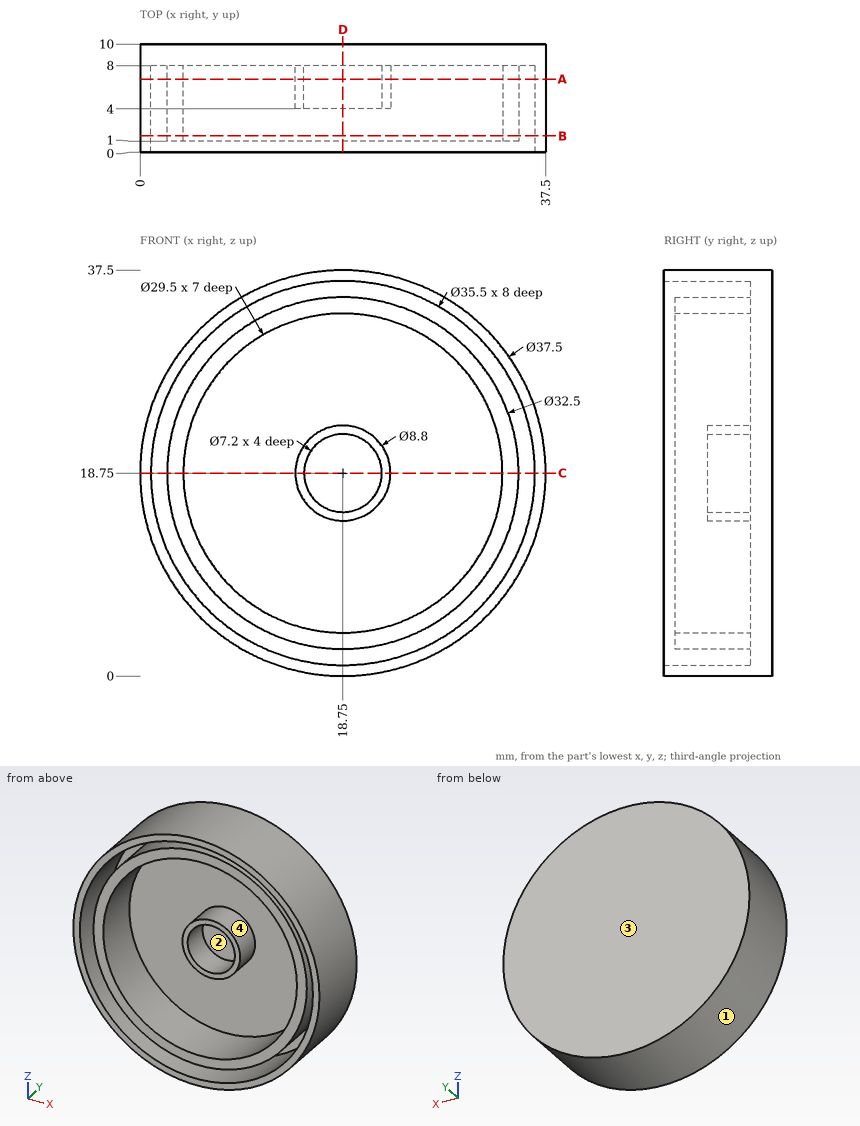
The drawing under review shows one solid part. Ordinate dimensions are in mm from its lowest x, y, z. Coordinates: 2 decimals unless noted, no trailing zeros. Write each loop counter-clockwise with the first axis right and the second up, starting at its lowest first coordinate (ties: lowest second). Pieces come first, ordered by that corner, then holes. Notation, with made-up numbers: M 62,-18 L 103,-18 A25 ccw 103,-1 Z; hole C 81,44.5 d5. An arc over 180 degrees is marked long. Answer as a JSON object with one key per item and string values.
Item 1: Add section D-D, the plane x = 18.75. Give the boundary of the cut face in (y, z).
Outcome:
{"outline": "M 0,0 L 10,0 L 10,37.5 L 0,37.5 L 0,36.5 L 8,36.5 L 8,35 L 1,35 L 1,33.5 L 8,33.5 L 8,23.15 L 4,23.15 L 4,22.35 L 8,22.35 L 8,15.15 L 4,15.15 L 4,14.35 L 8,14.35 L 8,4 L 1,4 L 1,2.5 L 8,2.5 L 8,1 L 0,1 Z"}
Item 2: Wall thickness on probe 1 along Z at (x, y) = (18.75, 3); probe 2 along Z at (x, y) = (18.75, 5.5); probe 3 along X at (y, z) = (5.25, 16.5): over which ranges is each line inside the solid? List them lowest first.
Outcome:
{"probe 1": "0 to 1, 2.5 to 4, 33.5 to 35, 36.5 to 37.5", "probe 2": "0 to 1, 2.5 to 4, 14.35 to 15.15, 22.35 to 23.15, 33.5 to 35, 36.5 to 37.5", "probe 3": "0.14 to 1.14, 2.66 to 4.17, 14.97 to 15.94, 21.56 to 22.53, 33.33 to 34.84, 36.36 to 37.36"}
Item 3: Add section B-B, the plane y = 1.5. Give the boundary of the cut face in (x, z).
Outcome:
{"outline": "C 18.75,18.75 d37.5; C 18.75,18.75 d32.5; hole C 18.75,18.75 d35.5; hole C 18.75,18.75 d29.5"}
Item 4: Add section C-C, the plane z = 18.75. Give the boundary of the cut face in (x, y), and give its area (3 significant figures).
Outcome:
{"outline": "M 0,0 L 1,0 L 1,8 L 2.5,8 L 2.5,1 L 4,1 L 4,8 L 14.35,8 L 14.35,4 L 15.15,4 L 15.15,8 L 22.35,8 L 22.35,4 L 23.15,4 L 23.15,8 L 33.5,8 L 33.5,1 L 35,1 L 35,8 L 36.5,8 L 36.5,0 L 37.5,0 L 37.5,10 L 0,10 Z", "area": "118 mm²"}
Item 5: Add section A-A, the plane y = 6.75. Give the boundary of the cut face in (x, z).
Outcome:
{"outline": "C 18.75,18.75 d37.5; C 18.75,18.75 d32.5; C 18.75,18.75 d8.8; hole C 18.75,18.75 d35.5; hole C 18.75,18.75 d29.5; hole C 18.75,18.75 d7.2"}
Item 6: Insertion check: pin 1 Ø4 at (y, z) = (1.5, 29.5) entering from -X; pin 2 Ø4 at (y, z) = (5.5, 5) entering from -X; pin 3 Ø9.5 at (x, z) = (20.5, 19.5) entering from -Y. Each pin has a flat end and moves straight along its axis. Give the tip position at first contact, or say it passes through.
Outcome:
{"pin 1": "x = 2.17", "pin 2": "x = 4.14", "pin 3": "y = 4"}
Item 7: Draft analysis for pull direction X (two halves, no side actions). For the marked faces 1, 2, 3 and 4, state which applies: pulls with the +X half, pulls with the -X half, needs draft (parallel to the pull), parting line crosses it, or undercut.
Outcome:
{"face 1": "parting line crosses it", "face 2": "undercut", "face 3": "needs draft", "face 4": "undercut"}
